Build history of the part. All positions in model axes, mm. Face numbers are marked on the shaded views. A direction names the side the tool comes from. Give positions to 0.01 mm unless a question says otherwise; leave off trailing zeros. Loops run counter-clockwise (first coordinate to the right, second up) from the corner with the lowest first, then second, coordinate; pieces in that order, holes last. Notation, with made-up numbers: (29.25, -6.75) -> (33.25, -6.75) arc R28 cw to (33.25, 28.25) -> close; hole circle Ø9 at (54.5, 39). An arc over 180 degrees is marked (long way). Answer as a JSON object with one key per item and string values. Group by question number.
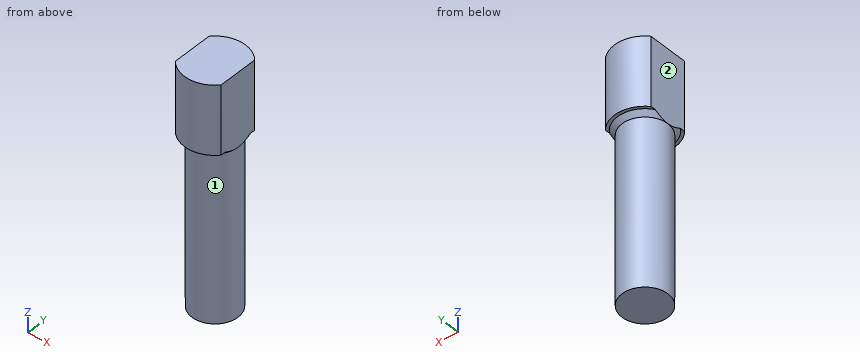
from build123d import *

# Parameters (mm, degrees)
SKETCH_1_R          = 15
EXTRUDE_1_DEPTH     = 112
SKETCH_2_R          = 20
EXTRUDE_2_DEPTH     = 45
CHAMFER_1_SIZE      = 3
SKETCH_3_W          = 15.452934815
SKETCH_3_H          = 42.066322552
CUT_EXTRUDE_3_DEPTH = 160.527427109


with BuildPart() as part:
    # Эскиз1 → Вытянуть1 (new body)
    with BuildSketch(Plane.XY):
        Circle(SKETCH_1_R)
    extrude(amount=EXTRUDE_1_DEPTH)

    # Эскиз2 → Вытянуть2 (add)
    with BuildSketch(Plane.XY.offset(112)):
        with Locations(Location((0, 0, 0), (0, 0, 180))):
            Circle(SKETCH_2_R)
    extrude(amount=EXTRUDE_2_DEPTH)

    # Фаска1
    chamfer_1_edges = [part.edges().sort_by_distance(p)[0] for p in [
        (-15, 0, 112),
    ]]
    chamfer(chamfer_1_edges, length=CHAMFER_1_SIZE)

    # Эскиз3 → Вытянуть3 (cut, through all)
    with BuildSketch(Plane.XY.offset(157)):
        with Locations((22.726467408, -0.268280118)):
            Rectangle(SKETCH_3_W, SKETCH_3_H)
        with Locations((-22.726467408, -0.268280118)):
            Rectangle(SKETCH_3_W, SKETCH_3_H)
    extrude(amount=-CUT_EXTRUDE_3_DEPTH, mode=Mode.SUBTRACT)


solid = part.part
(1) Probe line 1 along Z through (x, y) = (-12.5, -15.5); line 2 along X through (y, z) = (8.5, 96); line 3 along Y through (x, z) = (-10, 79). List the from-to ranges inside material, lowest first. Write a range as [from, to].
(2) Saw through at C-C on z = 116. List the corners of the cut face in (x, y).
(3) Pin check, flat tips, straight feed: pin 1 (12 mm diameter, centred on x = -7, z = 23.5, fed in from +Y); pin 2 (3 mm diameter, centred on y = 11, z = 57, fed in from +X). Stop position of each tip, or through.
(4) Saw through at A-A on x = 0. List the corners of the cut face in (y, z), plus the area to 3 significant figures.
(5) 3-axis set-ups, long thin cutter, end or side, ignore diameter. For the marked faces 1 and 2: which of +Z, -Z, +X, -X, +Y, -Y reach the whole face in a straight line?
(6) Saw through at B-B on z = 31. List the corners of the cut face in (x, y).
Calculated:
{
 "1": {"line 1": "z = [112, 157]", "line 2": "x = [-12.36, 12.36]", "line 3": "y = [-11.18, 11.18]"},
 "2": {"outline": "(-15, -13.23) arc R20 ccw to (15, -13.23) -> (15, 13.23) arc R20 ccw to (-15, 13.23) -> close"},
 "3": {"pin 1": "stops at y = 14.97", "pin 2": "stops at x = 11.61"},
 "4": {"outline": "(-20, 112) -> (-18, 112) -> (-15, 109) -> (-15, 0) -> (15, 0) -> (15, 109) -> (18, 112) -> (20, 112) -> (20, 157) -> (-20, 157) -> close", "area": "5,170 mm^2"},
 "5": {"face 1": "-Z", "face 2": "+Z, -Z, -X, +Y, -Y"},
 "6": {"outline": "circle Ø30 at (0, 0)"}
}
